from build123d import *

# Parameters (mm, degrees)
F1_DEPTH = 30
F0_R     = 20
F2_DEPTH = 12
F0_R_2   = 10
F3_DEPTH = 28


with BuildPart() as f1:
    # F0 (on Front) → F1 (new body)
    with BuildSketch(Plane.XZ):
        Polygon((-44, 0.63053), (-44, -29.36947), (-20, -29.36947), (-20, -14.36947), (20, -14.36947), (20, -29.36947), (44, -29.36947), (44, 0.63053), align=None)
    extrude(amount=-F1_DEPTH)

    # F0 (on Front) → F2 (join)
    with BuildSketch(Plane.XZ):
        Polygon((-44, 0.63053), (-44, -29.36947), (-20, -29.36947), (-20, -14.36947), (20, -14.36947), (20, -29.36947), (44, -29.36947), (44, 0.63053), align=None)
        with BuildLine():
            Line((-44, 40.63053), (-44, 0.63053))
            Line((-44, 0.63053), (44, 0.63053))
            Line((44, 0.63053), (44, 40.63053))
            ThreePointArc((44, 40.63053), (0, 84.63053), (-44, 40.63053))
        make_face()
        with Locations((0, 40.63053)):
            Circle(F0_R, mode=Mode.SUBTRACT)
    extrude(amount=-F2_DEPTH)

    # F0 (on Front) → F3 (join)
    with BuildSketch(Plane.XZ):
        with Locations((0, 40.63053)):
            Circle(F0_R)
        with Locations((0, 40.63053)):
            Circle(F0_R_2, mode=Mode.SUBTRACT)
    extrude(amount=-F3_DEPTH)


solid = f1.part
Source: CAD feature listing. Evaluate the final solid. Frame: model axes, mm. A direction names the side the tool comes from. Coordinates: 2 decimals unless noted, no trailing zeros. Order: outer loops, then holes, each group sorted by start corner. A loop starts at its lowest first (then second) coordinate and runs counter-clockwise, first axis right, second up. Notation, with made-up numbers: M -5,36.5 L 48,36.5 A30 cw 48,69.5 Z; hole C 12.25,40 d4. An arc over 180 degrees is marked long. Write each question's results on one line, items separated by ' | '. Start each with the question number.
Item 1: Cut plane D-D (z = 13.5). Return loops of the section in (x, y).
Item 2: Cut plane C-C (y = 7.25). Return loops of the section in (x, z), and give its area (3 significant figures).
Item 3: Line query: probe 1 along Z at (x, y) = (0, 18.5); probe 2 along Z at (x, y) = (0, 5.5); probe 3 along X at (y, z) = (24, -15). Output: solid intervals per line, ascending.
Item 4: First-contact query: pin 1 Ø2 at (x, z) = (23.5, 25.5) entering from -Y; pin 2 Ø4 at (x, y) = (-2, 25.5) entering from +Z; pin 3 Ø3 at (y, z) = (15.5, 38.5) entering from +X; pin 4 Ø12 at (x, z) = (-10, 72) entering from +Y. Flat tips, straight axial feed; report the tip coordinate or a pass-through.
Item 5: Set-up query: faces 5 (the face through (1, 21, 0.631)), 6 (the face through (20, 15, -22)), 7 (the face through (4, 28, 50)), 8 (the face through (-4.3, 19.9, 21.1)). Return all of +Z, -Z, +X, -X, +Y, -Y with unobstructed straight access to the full face (end or side cutting, diameter ignored); none if empty.
Item 6: Draft query along X for faces 1 (the face through (0, 15, -14.369)), 2 (the face through (-20, 15, -22)), 3 (the face through (-44, 11, -2)), 4 (the face through (0.97, 5.92, 84.62)). Return one class per face: pulls with the +X half, pulls with the -X half, needs draft (parallel to the pull), parting line crosses it, or undercut.
Item 7: Cut plane A-A (x = 0). Return loops of the section in (y, z).
Item 8: Cut plane B-B (y = 18). Return loops of the section in (x, z).
Checked values:
1) outline: M -44,0 L 44,0 L 44,12 L -44,12 Z
2) outline: M -44,-29.37 L -20,-29.37 L -20,-14.37 L 20,-14.37 L 20,-29.37 L 44,-29.37 L 44,40.63 A44 ccw -44,40.63 Z; hole C 0,40.63 d20 | area: 8,290 mm2
3) probe 1: z = -14.37 to 0.63, 20.63 to 30.63, 50.63 to 60.63 | probe 2: z = -14.37 to 30.63, 50.63 to 84.63 | probe 3: x = -44 to -20, 20 to 44
4) pin 1: stops at y = 0 | pin 2: stops at z = 60.63 | pin 3: stops at x = 19.99 | pin 4: stops at y = 12
5) face 5: +X, -X, +Y | face 6: -Z, +Y, -Y | face 7: +Z, +X, -X, +Y | face 8: +Y
6) face 1: undercut | face 2: undercut | face 3: pulls with the -X half | face 4: parting line crosses it
7) outline: M 0,-14.37 L 30,-14.37 L 30,0.63 L 12,0.63 L 12,20.63 L 28,20.63 L 28,30.63 L 0,30.63 Z; M 0,50.63 L 28,50.63 L 28,60.63 L 12,60.63 L 12,84.63 L 0,84.63 Z
8) outline: M -44,-29.37 L -20,-29.37 L -20,-14.37 L 20,-14.37 L 20,-29.37 L 44,-29.37 L 44,0.63 L -44,0.63 Z; C 0,40.63 d40; hole C 0,40.63 d20
